```python
from build123d import *

# Parameters (mm, degrees)
SKETCH1_R           = 2.5
BOSS_EXTRUDE1_DEPTH = 2


with BuildPart() as part:
    # Sketch1 → Boss-Extrude1 (new body)
    with BuildSketch(Plane.XY):
        with BuildLine():
            Line((245.25, -5.629165125), (343.630404909, -62.429118382))
            ThreePointArc((343.630404909, -62.429118382), (350.130404909, -62.429118382), (353.380404909, -56.799953257))
            Line((353.380404909, -56.799953257), (353.380404909, 56.799953257))
            ThreePointArc((353.380404909, 56.799953257), (350.130404909, 62.429118382), (343.630404909, 62.429118382))
            Line((343.630404909, 62.429118382), (245.25, 5.629165125))
            ThreePointArc((245.25, 5.629165125), (242, 0), (245.25, -5.629165125))
        make_face()
        with Locations((248.5, 0)):
            Circle(SKETCH1_R, mode=Mode.SUBTRACT)
        with Locations((346.880404909, -56.799953257)):
            Circle(SKETCH1_R, mode=Mode.SUBTRACT)
        with Locations((346.880404909, 56.799953257)):
            Circle(SKETCH1_R, mode=Mode.SUBTRACT)
        with BuildLine():
            Line((264.5, 1.732050808), (337.380404909, 43.809572201))
            ThreePointArc((337.380404909, 43.809572201), (339.380404909, 43.809572201), (340.380404909, 42.077521393))
            Line((340.380404909, 42.077521393), (340.380404909, -42.077521393))
            ThreePointArc((340.380404909, -42.077521393), (339.380404909, -43.809572201), (337.380404909, -43.809572201))
            Line((337.380404909, -43.809572201), (264.5, -1.732050808))
            ThreePointArc((264.5, -1.732050808), (263.5, 0), (264.5, 1.732050808))
        make_face(mode=Mode.SUBTRACT)
    extrude(amount=BOSS_EXTRUDE1_DEPTH)


solid = part.part
```
Work out the finished part from the listing and answer in its coordinate system (mm). A direction names the side the tool comes from. Give positions to 0.01 mm unless a question says otherwise; leave off trailing zeros. Loops run counter-clockwise (first coordinate to the right, second up) from the corner with the lowest first, then second, coordinate; pieces in that order, holes last. Notation, with made-up numbers: M 65.5,15.5 L 92.5,15.5 A24 cw 92.5,52.5 Z; hole C -21.5,74 d1. An arc over 180 degrees is marked long. One line per item, written item: value. Start each with the question number.
1. Which of the six approach directions +Z, -Z, +X, -X, +Y, -Y give full straight-line access (tool end or side, diameter ignored) to faces 4 (the face through (300.43, 22.476, 0.986)), 5 (the face through (302, 24, 0))?
2. Determine the mould class of faces 1 (the face through (345.04, -55.11, 0.99)), 2 (the face through (295.129, 34.427, 0.986)), 3 (the face through (242, 0, 1)) for opening direction Y: released by +Y, released by -Y, zero draft, split by the parting line, or undercut.
3. Find section C-C (x = 304.5). Give the vertices of the cut face in (y, z), and give its area (3 significant figures).
4. Find section B-B (z = 0.5). Give the vertices of the cut face in (x, y), and give its area (3 significant figures).
5. This flat-tipped pin is pushed along its axis until it touches: P1, Ø1, axis at y = 11, z = 1, coming from the -X side. Where does it stop, or does it pass through?
6. Find section A-A (y = 0). Give the vertices of the cut face in (x, z).
7. Find section D-D (y = 31). Give the vertices of the cut face in (x, z).
8. Find the intervals of material crossed by probe 1 along Y at (x, z) = (348, 1.3); probe 2 along Y at (x, z) = (313, 1.2); probe 3 along Y at (x, z) = (274.5, 0.2), in increasing order.
Reported:
1. face 4: +Z, -Z
1. face 5: -Z, +X, -X, +Y, -Y
2. face 1: undercut
2. face 2: released by +Y
2. face 3: split by the parting line
3. outline: M -39.84,0 L -24.83,0 L -24.83,2 L -39.84,2 Z; M 24.83,0 L 39.84,0 L 39.84,2 L 24.83,2 Z
3. area: 60.0 mm²
4. outline: M 245.25,-5.63 L 343.63,-62.43 A6.5 ccw 353.38,-56.8 L 353.38,56.8 A6.5 ccw 343.63,62.43 L 245.25,5.63 A6.5 ccw Z; hole C 248.5,0 d5; hole M 264.5,-1.73 L 337.38,-43.81 A2 ccw 340.38,-42.08 L 340.38,42.08 A2 ccw 337.38,43.81 L 264.5,1.73 A2 ccw Z; hole C 346.88,-56.8 d5; hole C 346.88,56.8 d5
4. area: 4,290 mm²
5. P1: stops at x = 253.69
6. outline: M 242,0 L 246,0 L 246,2 L 242,2 Z; M 251,0 L 263.5,0 L 263.5,2 L 251,2 Z; M 340.38,0 L 353.38,0 L 353.38,2 L 340.38,2 Z
7. outline: M 289.19,0 L 315.19,0 L 315.19,2 L 289.19,2 Z; M 340.38,0 L 353.38,0 L 353.38,2 L 340.38,2 Z
8. probe 1: y = -63.2 to -59.04, -54.56 to 54.56, 59.04 to 63.2
8. probe 2: y = -44.74 to -29.73, 29.73 to 44.74
8. probe 3: y = -22.52 to -7.51, 7.51 to 22.52
